Geometry check sheet. Reference: the model listing, model coordinates, mm. Give positions to 0.01 mm unless a question says otherwise; leave off trailing zeros. Write each loop counter-clockwise with the first axis right and the second up, starting at its lowest first coordinate (ties: lowest second). Pieces come first, ordered by that corner, then holes. Notation, with made-up numbers: (-4, -38) - (39, -38) arc R9 ccw to (39, -31) - close; hole circle Ø9 at (-14.5, -9.75). An arc over 180 degrees is marked (long way). One line per question, with ' | ' between items. Start each with the question number.
Q1. Section check B-B on z = 5.5. Record the boundary of the cut face in (x, y) (3 decimals).
Q2. Section check D-D on y = 29.5. Record the boundary of the cut face in (x, z).
Q3. Release check for a two-part mould opening along X. For faces 1 (the face through (79, 33, 0)), 2 (the face through (53.41, 52.47, 4.93)), 3 (the face through (207.879, 2, 5)) record: +X half, -X half, draft (parallel to the pull), parting line (faces both ways), or undercut.
Q4. Section check C-C on x = 181. Record the boundary of the cut face in (y, z), and give its area (3 significant figures).
Q5. Section check A-A on y = 46. Record the boundary of the cut face in (x, z), and give its area (3 significant figures).
Q6. Thickness scan on L1, parallel to X at y = 49.5, z = 1; L2, parallel to X at y = 48, z = 2.75; L3, parallel to Y at x = 59, z = 5.5. Record the ranges inside material, lowest first. Write a range as [from, to].
Q7. Gauge pin test, flat ends, axial feed: P1, Ø3, axis at y = 59, z = 7.5, coming from the -X side; P2, Ø5, axis at y = 16.5, z = 2, coming from the -X side; P3, Ø2, axis at x = 142, y = 46, coming from the +Z side. Record the tip position at first contact, or that the pin passes through.
```python
from build123d import *

# Parameters (mm, degrees)
ESQUISSE1_R        = 10.125
BOSS_EXTRU_1_DEPTH = 10


with BuildPart() as part:
    # Esquisse1 → Boss.-Extru.1 (new body)
    with BuildSketch(Plane.XY):
        with BuildLine():
            Line((0, 0), (207.878588044, 0))
            Line((207.878588044, 0), (207.878588044, 5))
            Line((207.878588044, 5), (81.20130317, 78.137164522))
            ThreePointArc((81.20130317, 78.137164522), (57.130536246, 82.902959743), (36.932524958, 68.969009678))
            Line((36.932524958, 68.969009678), (0, 5))
            Line((0, 5), (0, 0))
        make_face()
        with Locations((63.524775179, 52.028138149)):
            Circle(ESQUISSE1_R, mode=Mode.SUBTRACT)
    extrude(amount=BOSS_EXTRU_1_DEPTH)


solid = part.part
```
Working result:
1) outline: (0, 0) - (207.879, 0) - (207.879, 5) - (81.201, 78.137) arc R31.53 ccw to (36.933, 68.969) - (0, 5) - close; hole circle Ø20.25 at (63.525, 52.028)
2) outline: (14.15, 0) - (165.44, 0) - (165.44, 10) - (14.15, 10) - close
3) face 1: draft | face 2: undercut | face 3: +X half
4) outline: (0, 0) - (20.52, 0) - (20.52, 10) - (0, 10) - close | area: 205 mm2
5) outline: (23.67, 0) - (55.39, 0) - (55.39, 10) - (23.67, 10) - close; (71.66, 0) - (136.86, 0) - (136.86, 10) - (71.66, 10) - close | area: 969 mm2
6) L1: x = [25.69, 53.72], [73.33, 130.8] | L2: x = [24.83, 54.24], [72.81, 133.4] | L3: y = [0, 42.97], [61.09, 83.23]
7) P1: stops at x = 30.31 | P2: stops at x = 5.2 | P3: passes through
